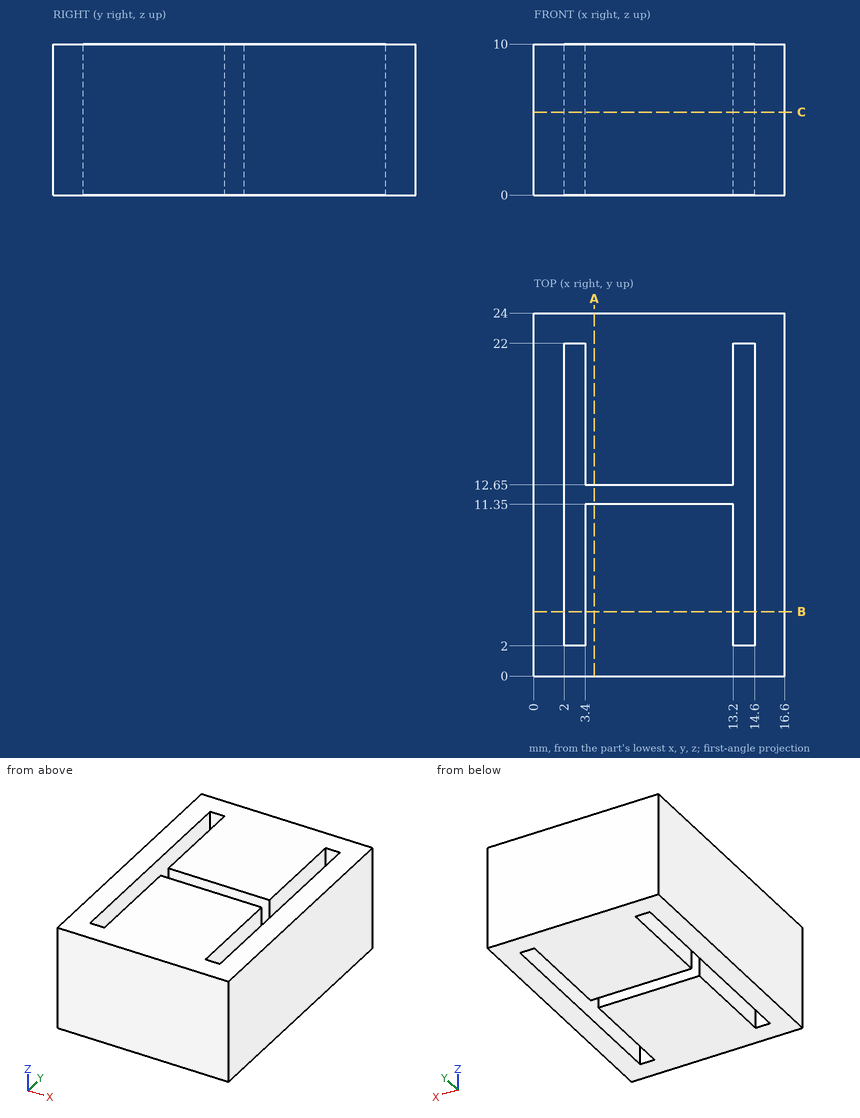
Geometry check sheet. Reference: drawing and pictorial views, mm from the part's lowest x, y, z. Coordinates: 2 decimals unless noted, no trailing zeros. Write each loop counter-clockwise with the first axis right and the second up, starting at its lowest first coordinate (ties: lowest second). Pieces come first, ordered by that corner, then holes. Notation, with made-up numbers: M 34.5,38 L 55.5,38 A22 cw 55.5,65 Z; hole C 85,11.25 d7. An arc over 180 degrees is marked long. Use one line per item in the form item = value.
Item 1: Material ranges on L1, parallel to X at y = 7.5, z = 3.5; L2, parallel to Y at x = 13.5, z = 2.75; L3, parallel to Y at x = 6.5, z = 5.5, recorded low to high. Write a range as from..to.
Answer below:
L1 = 0..2, 3.4..13.2, 14.6..16.6
L2 = 0..2, 22..24
L3 = 0..11.35, 12.65..24
Item 2: Sectioned sample at B-B, the plane y = 4.25. Record the cut outline in (x, z).
Answer below:
outline = M 0,0 L 2,0 L 2,10 L 0,10 Z; M 3.4,0 L 13.2,0 L 13.2,10 L 3.4,10 Z; M 14.6,0 L 16.6,0 L 16.6,10 L 14.6,10 Z
Item 3: Sectioned sample at C-C, the plane z = 5.5. Record the cut outline in (x, y).
Answer below:
outline = M 0,0 L 16.6,0 L 16.6,24 L 0,24 Z; hole M 2,2 L 3.4,2 L 3.4,11.35 L 13.2,11.35 L 13.2,2 L 14.6,2 L 14.6,22 L 13.2,22 L 13.2,12.65 L 3.4,12.65 L 3.4,22 L 2,22 Z
Item 4: Sectioned sample at A-A, the plane x = 4. Record the cut outline in (y, z).
Answer below:
outline = M 0,0 L 11.35,0 L 11.35,10 L 0,10 Z; M 12.65,0 L 24,0 L 24,10 L 12.65,10 Z
Item 5: Gauge pin test, flat end, axial feed: pin 1 Ø2 at (y, z) = (11.5, 5) entering from -X. Record the tip position at first contact, or that the pin passes through.
Answer below:
pin_1 = 0
